```python
from build123d import *

# Parameters (mm, degrees)
SKETCH1_W           = 24
SKETCH1_H           = 24
SKETCH1_R           = 0.75
BOSS_EXTRUDE1_DEPTH = 5
FILLET1_R           = 5
CUT_EXTRUDE1_DEPTH  = 10


with BuildPart() as part:
    # Sketch1 → Boss-Extrude1 (new body)
    with BuildSketch(Plane.XY):
        Rectangle(SKETCH1_W, SKETCH1_H)
        with Locations((-7.5, 7.5)):
            Circle(SKETCH1_R, mode=Mode.SUBTRACT)
        with Locations((7.5, 7.5)):
            Circle(SKETCH1_R, mode=Mode.SUBTRACT)
        with Locations((7.5, -7.5)):
            Circle(SKETCH1_R, mode=Mode.SUBTRACT)
        with Locations((-7.5, -7.5)):
            Circle(SKETCH1_R, mode=Mode.SUBTRACT)
    extrude(amount=BOSS_EXTRUDE1_DEPTH)

    # Fillet1
    fillet1_edges = [part.edges().sort_by_distance(p)[0] for p in [
        (-12, 12, 2.5),
        (12, 12, 2.5),
    ]]
    fillet(fillet1_edges, radius=FILLET1_R)

    # Sketch2 → Cut-Extrude1 (cut)
    with BuildSketch(Plane.XY.offset(5)):
        Polygon((-2, -12), (-2, -10.5), (-3, -10.5), (-3, -8), (-2, -8), (-2, -7), (2, -7), (2, -8), (3, -8), (3, -10.5), (2, -10.5), (2, -12), align=None)
    extrude(amount=-CUT_EXTRUDE1_DEPTH, mode=Mode.SUBTRACT)


solid = part.part
```
Geometry check sheet. Reference: the model listing, model coordinates, mm. A direction names the side the tool comes from. Give positions to 0.01 mm unless a question says otherwise; leave off trailing zeros. Write each loop counter-clockwise with the first axis right and the second up, starting at its lowest first coordinate (ties: lowest second). Pieces come first, ordered by that corner, then holes. Notation, with made-up numbers: (45, 36) -> (67, 36) arc R32 ccw to (67, 69) -> close; hole circle Ø10 at (-9, 8). An arc over 180 degrees is marked (long way). Use one line per item in the form item = value.
Item 1: Access from +Z, -Z, +X, -X, +Y, -Y to the whole of each face (thin tool, end or side, straight path). Record for faces 1 (the flat face through (2, -11, 3)), 2 (the flat face through (7, -12, 2)), 3 (the flat face through (-2.5, -10.5, 2.5)).
Results list:
face_1 = +Z, -Z, -Y
face_2 = +Z, -Z, +X, -X, -Y
face_3 = +Z, -Z
Item 2: Depth check by flat-ended pin: pin 1 Ø2 at (x, z) = (-0.5, 1.5) entering from -Y. Enter the tip coordinate at first touch or a pass-through.
Results list:
pin_1 = -7
Item 3: Sectioned sample at B-B on z = 2.5. Enter the section's corners in (x, y), plus the area to 3 significant figures.
Results list:
outline = (-12, -12) -> (-2, -12) -> (-2, -10.5) -> (-3, -10.5) -> (-3, -8) -> (-2, -8) -> (-2, -7) -> (2, -7) -> (2, -8) -> (3, -8) -> (3, -10.5) -> (2, -10.5) -> (2, -12) -> (12, -12) -> (12, 7) arc R5 ccw to (7, 12) -> (-7, 12) arc R5 ccw to (-12, 7) -> close; hole circle Ø1.5 at (-7.5, -7.5); hole circle Ø1.5 at (-7.5, 7.5); hole circle Ø1.5 at (7.5, -7.5); hole circle Ø1.5 at (7.5, 7.5)
area = 533 mm2
Item 4: Sectioned sample at C-C on x = 7.5. Enter the section's corners in (y, z), plus the area to 3 significant figures.
Results list:
outline = (-12, 0) -> (-8.25, 0) -> (-8.25, 5) -> (-12, 5) -> close; (-6.75, 0) -> (6.75, 0) -> (6.75, 5) -> (-6.75, 5) -> close; (8.25, 0) -> (11.97, 0) -> (11.97, 5) -> (8.25, 5) -> close
area = 105 mm2
Item 5: Sectioned sample at A-A on y = -7.5. Enter the section's corners in (x, z).
Results list:
outline = (-12, 0) -> (-8.25, 0) -> (-8.25, 5) -> (-12, 5) -> close; (-6.75, 0) -> (-2, 0) -> (-2, 5) -> (-6.75, 5) -> close; (2, 0) -> (6.75, 0) -> (6.75, 5) -> (2, 5) -> close; (8.25, 0) -> (12, 0) -> (12, 5) -> (8.25, 5) -> close
Item 6: Scan lines: line 1 (Y direction, x = -2.25, z = 0.4); line 2 (X direction, y = -9, z = 3.6); line 3 (Y direction, x = -7.5, z = 2.7). Record each from-to range of solid material in increasing order.
Results list:
line_1 = -12 to -10.5, -8 to 12
line_2 = -12 to -3, 3 to 12
line_3 = -12 to -8.25, -6.75 to 6.75, 8.25 to 11.97
Item 7: Sectioned sample at D-D on y = 7.5. Enter the section's corners in (x, z).
Results list:
outline = (-11.97, 0) -> (-8.25, 0) -> (-8.25, 5) -> (-11.97, 5) -> close; (-6.75, 0) -> (6.75, 0) -> (6.75, 5) -> (-6.75, 5) -> close; (8.25, 0) -> (11.97, 0) -> (11.97, 5) -> (8.25, 5) -> close
Item 8: Mould release check, pull along Y, two halves, no side actions. Record for faces 4 (the cylindrical face through (6.75, -7.47, 2.46)), 5 (the flat face through (0, -7, 3)), 6 (the flat face through (-2, -11, 3)), 7 (the flat face through (2.5, -8, 2.5)): released by +Y, released by -Y, zero draft, split by the parting line, or undercut.
Results list:
face_4 = undercut
face_5 = released by -Y
face_6 = zero draft
face_7 = undercut
